from build123d import *

# Parameters (mm, degrees)
SKETCH_1_W      = 45.369381955
SKETCH_1_H      = 45
SKETCH_1_R      = 1
SKETCH_1_W_2    = 5.6
SKETCH_1_H_2    = 5.6
EXTRUDE_1_DEPTH = 0.6
SKETCH_2_R      = 3.5
SKETCH_2_R_2    = 1
SKETCH_2_R_3    = 0.994011389
EXTRUDE_2_DEPTH = 1


with BuildPart() as part:
    # Эскиз1 → Бобышка-Вытянуть1 (new body)
    with BuildSketch(Plane(origin=(0, 0, 0), x_dir=(1, 0, 0), z_dir=(0, 1, 0))):
        with Locations((22.684690978, 22.5)):
            Rectangle(SKETCH_1_W, SKETCH_1_H)
        with Locations((6.737781955, 41.202537594)):
            Circle(SKETCH_1_R, mode=Mode.SUBTRACT)
        with Locations((40.537781955, 41.202537594)):
            Circle(SKETCH_1_R, mode=Mode.SUBTRACT)
        with Locations((40.537781955, 6.202537594)):
            Circle(SKETCH_1_R, mode=Mode.SUBTRACT)
        with Locations((6.737781955, 6.202537594)):
            Circle(SKETCH_1_R, mode=Mode.SUBTRACT)
        with Locations((15.437781955, 37.402537594)):
            Rectangle(SKETCH_1_W_2, SKETCH_1_H_2, mode=Mode.SUBTRACT)
        with Locations((15.437781955, 31.302537594)):
            Rectangle(SKETCH_1_W_2, SKETCH_1_H_2, mode=Mode.SUBTRACT)
        with Locations((15.437781955, 25.202537594)):
            Rectangle(SKETCH_1_W_2, SKETCH_1_H_2, mode=Mode.SUBTRACT)
        with Locations((15.437781955, 19.102537594)):
            Rectangle(SKETCH_1_W_2, SKETCH_1_H_2, mode=Mode.SUBTRACT)
        with Locations((15.437781955, 13.002237594)):
            Rectangle(SKETCH_1_W_2, SKETCH_1_H_2, mode=Mode.SUBTRACT)
        with Locations((31.837781955, 10.002237594)):
            Rectangle(SKETCH_1_W_2, SKETCH_1_H_2, mode=Mode.SUBTRACT)
        with Locations((31.837781955, 16.102237594)):
            Rectangle(SKETCH_1_W_2, SKETCH_1_H_2, mode=Mode.SUBTRACT)
        with Locations((31.837781955, 22.087504722)):
            Rectangle(SKETCH_1_W_2, SKETCH_1_H_2, mode=Mode.SUBTRACT)
        with Locations((31.837781955, 28.302237594)):
            Rectangle(SKETCH_1_W_2, SKETCH_1_H_2, mode=Mode.SUBTRACT)
        with Locations((31.837781955, 34.402237594)):
            Rectangle(SKETCH_1_W_2, SKETCH_1_H_2, mode=Mode.SUBTRACT)
    extrude(amount=EXTRUDE_1_DEPTH)

    # Эскиз2 → Бобышка-Вытянуть2 (add)
    with BuildSketch(Plane.XZ):
        with Locations((6.737781955, -6.202537594)):
            Circle(SKETCH_2_R)
        with Locations((6.737781955, -6.202537594)):
            Circle(SKETCH_2_R_2, mode=Mode.SUBTRACT)
        with Locations((40.537781955, -6.202537594)):
            Circle(SKETCH_2_R)
        with Locations((40.537781955, -6.202537594)):
            Circle(SKETCH_2_R_2, mode=Mode.SUBTRACT)
        with Locations((40.537781955, -41.202537594)):
            Circle(SKETCH_2_R)
        with Locations((40.537781955, -41.202537594)):
            Circle(SKETCH_2_R_3, mode=Mode.SUBTRACT)
        with Locations((6.737781955, -41.202537594)):
            Circle(SKETCH_2_R)
        with Locations((6.737781955, -41.202537594)):
            Circle(SKETCH_2_R_2, mode=Mode.SUBTRACT)
    extrude(amount=EXTRUDE_2_DEPTH)


solid = part.part
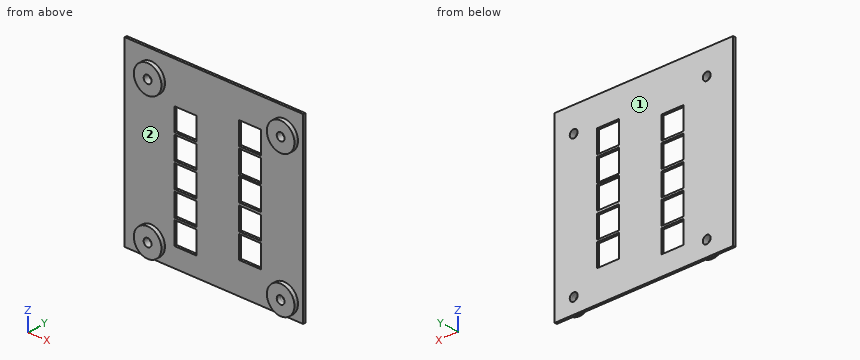
The model under review builds one solid part; all positions refer to its coordinate system, in mm. Face numbers are marked on the shaded views. Round coordinates to 2 decimals unless told otherwise and drop trailing zeros. Loops run counter-clockwise (first coordinate to the right, second up) from the corner with the lowest first, then second, coordinate; pieces in that order, holes last. Notation, with made-up numbers: M 11.5,-34 L 24.5,-34 A19 ccw 24.5,3 Z; hole C 40,86 d4. An arc over 180 degrees is marked long. Answer as CSV lines item,"result". Start each with the question number.
Item 1: Wall thickness on line 1 (X direction, y = 0.3, z = -35); line 2 (Z direction, x = 32, y = 0.5); line 3 (Z direction, x = 13, y = 0.2): over which ranges is each line inside the solid? List them lowest first. Write a range as [from, to].
Item 2: Consider section C-C (y = -0.65). Write out the cut boundary in (x, z).
Item 3: Consider section A-A (z = -27). Write out the cut boundary in (x, y), then the cut area to 3 significant figures.
Item 4: Consider section D-D (x = 41). State how many separate pieces and enclosed holes the cut face has, then the cut area to 3 significant figures.
Item 5: Consider section B-B (x = 30). Write out the cut boundary in (y, z).
Item 6: Insertion check: P1, Ø13.5, axis at x = 12, z = -32.5, coming from the -Y side; P2, Ø1.6, axis at x = 40.54, z = -41.2, coming from the -Y side. Each pin has a flat end and moves straight along its axis. Give the tip position at first contact, or say it passes through.
Item 7: Mouldability with a two-part tool opening along X and no side actions: class the marked faces 1 and 2 as released by +X, released by -X, zero draft, split by the parting line, or undercut.
Answer:
1,line 1,"x = [0, 12.64], [18.24, 29.04], [34.64, 45.37]"
1,line 2,"z = [-45, -37.2], [-31.6, -31.1], [-25.5, -24.89], [-19.29, -18.9], [-13.3, -12.8], [-7.2, 0]"
1,line 3,"z = [-45, -40.2], [-34.6, -34.1], [-28.5, -28], [-22.4, -21.9], [-16.3, -15.8], [-10.2, 0]"
2,outline,"C 6.74,-41.2 d7; C 6.74,-6.2 d7; C 40.54,-41.2 d7; C 40.54,-6.2 d7; hole C 6.74,-41.2 d2; hole C 6.74,-6.2 d2; hole C 40.54,-41.2 d1.99; hole C 40.54,-6.2 d2"
3,outline,"M 0,0 L 12.64,0 L 12.64,0.6 L 0,0.6 Z; M 18.24,0 L 29.04,0 L 29.04,0.6 L 18.24,0.6 Z; M 34.64,0 L 45.37,0 L 45.37,0.6 L 34.64,0.6 Z"
3,area,"20.5 mm^2"
4,separate pieces,"3"
4,enclosed holes,"0"
4,area,"35.2 mm^2"
5,outline,"M 0,-45 L 0.6,-45 L 0.6,-37.2 L 0,-37.2 Z; M 0,-31.6 L 0.6,-31.6 L 0.6,-31.1 L 0,-31.1 Z; M 0,-25.5 L 0.6,-25.5 L 0.6,-24.89 L 0,-24.89 Z; M 0,-19.29 L 0.6,-19.29 L 0.6,-18.9 L 0,-18.9 Z; M 0,-13.3 L 0.6,-13.3 L 0.6,-12.8 L 0,-12.8 Z; M 0,-7.2 L 0.6,-7.2 L 0.6,0 L 0,0 Z"
6,P1,"stops at y = -1"
6,P2,"passes through"
7,face 1,"zero draft"
7,face 2,"undercut"
